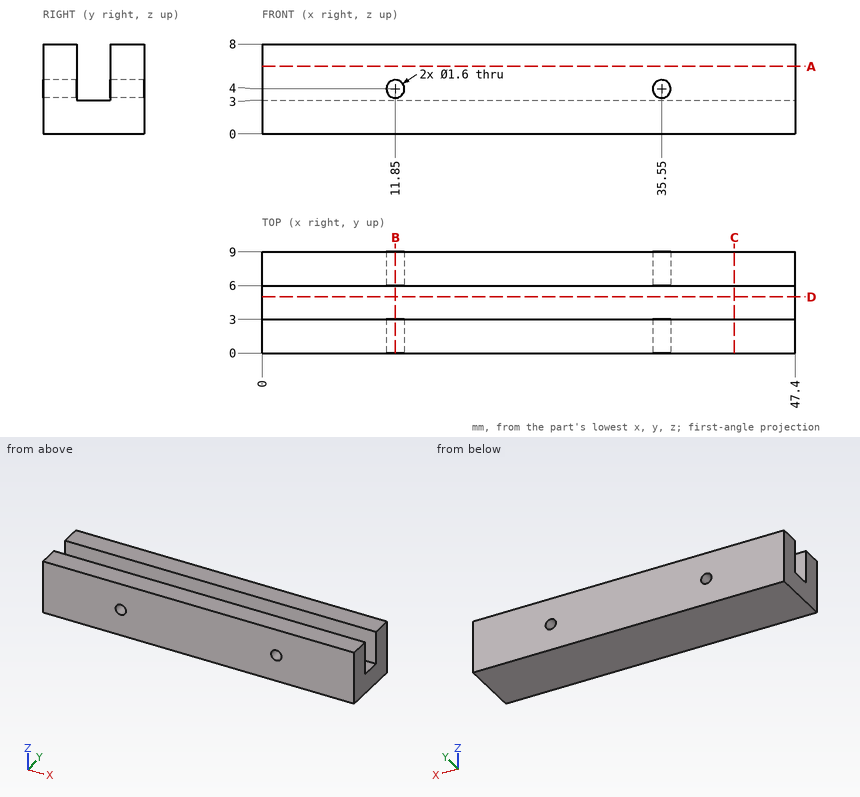
Design review of the part shown in the three views and the two pictorial views. Dimensions are in mm from the part's minimum x, y and z. Coordinates: 2 decimals unless noted, no trailing zeros. Loops run counter-clockwise (first coordinate to the right, second up) from the corner with the lowest first, then second, coordinate; pieces in that order, holes last. Notation, with made-up numbers: M -24.75,-5 L 7.25,-5 A22 cw 7.25,12 Z; hole C -7,1 d3. An arc over 180 degrees is marked long. Put each result on its own line as item: value. Start each with the question number.
Q1. Clearance check with flat-ended pins moving along their axes: pin 1 (4 mm diameter, centred on x = 18, z = 4, fed in from -Y); pin 2 (1.4 mm diameter, centred on x = 35.55, z = 4, fed in from +Y); pin 3 (2.5 mm diameter, centred on x = 35.5, y = 4.5, fed in from +Z). State where each tip first meets the part, or that it passes through.
Q2. Add section C-C (x = 42). Write out the cut boundary in (y, z).
Q3. Add section B-B (x = 11.85). Write out the cut boundary in (y, z).
Q4. Add section D-D (y = 5). Write out the cut boundary in (x, z).
Q5. Add section A-A (z = 6). Write out the cut boundary in (x, y).
Q6. Wall thickness on line 1 (X direction, y = 6.25, z = 4); line 2 (Y direction, x = 6.5, z = 3.5); line 3 (Z direction, x = 35.55, y = 1.05): over which ranges is each line inside the solid? List them lowest first.
Answers:
1. pin 1: stops at y = 0
1. pin 2: passes through
1. pin 3: stops at z = 3
2. outline: M 0,0 L 9,0 L 9,8 L 6,8 L 6,3 L 3,3 L 3,8 L 0,8 Z
3. outline: M 0,0 L 9,0 L 9,3.2 L 6,3.2 L 6,3 L 3,3 L 3,3.2 L 0,3.2 Z; M 0,4.8 L 3,4.8 L 3,8 L 0,8 Z; M 6,4.8 L 9,4.8 L 9,8 L 6,8 Z
4. outline: M 0,0 L 47.4,0 L 47.4,3 L 0,3 Z
5. outline: M 0,0 L 47.4,0 L 47.4,3 L 0,3 Z; M 0,6 L 47.4,6 L 47.4,9 L 0,9 Z
6. line 1: x = 0 to 11.05, 12.65 to 34.75, 36.35 to 47.4
6. line 2: y = 0 to 3, 6 to 9
6. line 3: z = 0 to 3.2, 4.8 to 8
